Design review of the part built by this model. Coordinates are the model's own, in mm. Round coordinates to 2 decimals unless told otherwise and drop trailing zeros. Write each loop counter-clockwise with the first axis right and the second up, starting at its lowest first coordinate (ties: lowest second). Pieces come first, ordered by that corner, then holes. Notation, with made-up numbers: (-33.75, -40) -> (-22.75, -40) arc R13 cw to (-22.75, -26) -> close; hole circle Ø1 at (40.5, 79). An arc over 180 degrees is marked (long way). Write item = value, one per line. Start each with the question number.
Item 1: To check wall thickness, follow L1, parallel to Y at x = 12.5, z = 0.2; L2, parallel to Y at x = 10, z = 0.45; L3, parallel to Y at x = 14, z = 0.3. State the ranges of each line that lie inside material, in increasing order.
Item 2: Add section C-C, the plane x = 18.5. State the section outline as (y, z) points, then the cut area to 3 significant figures.
Item 3: Add section D-D, the plane y = -52. State the section outline as (x, z) points.
Item 4: Add section B-B, the plane y = 0. State the section outline as (x, z) points.
Item 5: Add section A-A, the plane z = 0.3. State how many separate pieces and enclosed holes the cut face has, then the cut area to 3 significant figures.
Item 6: For pin 1 Ø1 at (y, z) = (-20, 2) entering from -X; pin 2 Ø0.6 at (x, z) = (19, 0.5) entering from -Y; pin 3 Ø0.6 at (x, z) = (-10, 1) entering from -Y, all flat-tipped, find the tip position at first contact; note any pin that passes through.
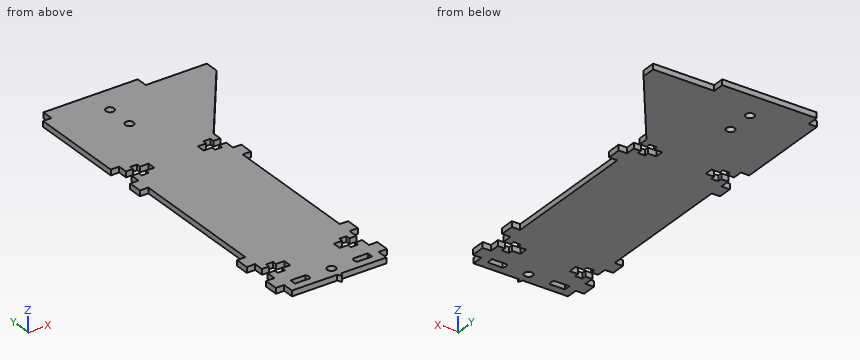
from build123d import *

# Parameters (mm, degrees)
SKETCH_1_R      = 1.5
EXTRUDE_1_DEPTH = 2


with BuildPart() as part:
    # 草图1 → 凸台-拉伸1 (new body)
    with BuildSketch(Plane.XY):
        Polygon((16.993865071, -34), (16.993865071, -84), (19.993865071, -84), (19.993865071, -89), (16.993865071, -89), (16.993865071, -92.5), (14.493865071, -92.5), (14.493865071, -91), (11.893865071, -91), (11.893865071, -92.5), (8.893865071, -92.5), (8.893865071, -95.5), (11.893865071, -95.5), (11.893865071, -97), (14.493865071, -97), (14.493865071, -95.5), (16.993865071, -95.5), (16.993865071, -99), (19.993865071, -99), (19.993865071, -104), (16.993865071, -104), (16.993865071, -108), (0.721190694, -108), (0, -109.5), (-0.721190694, -108), (-16.993865071, -108), (-16.993865071, -104), (-19.993865071, -104), (-19.993865071, -99), (-16.993865071, -99), (-16.993865071, -95.5), (-14.493865071, -95.5), (-14.493865071, -97), (-11.893865071, -97), (-11.893865071, -95.5), (-8.893865071, -95.5), (-8.893865071, -92.5), (-11.893865071, -92.5), (-11.893865071, -91), (-14.493865071, -91), (-14.493865071, -92.5), (-16.993865071, -92.5), (-16.993865071, -89), (-19.993865071, -89), (-19.993865071, -84), (-16.993865071, -84), (-16.993865071, -34), (-19.993865071, -34), (-19.993865071, -29), (-16.993865071, -29), (-16.993865071, -25.5), (-14.493865071, -25.5), (-14.493865071, -27), (-11.893865071, -27), (-11.893865071, -25.5), (-8.893865071, -25.5), (-8.893865071, -22.5), (-11.893865071, -22.5), (-11.893865071, -21), (-14.493865071, -21), (-14.493865071, -22.5), (-16.993865071, -22.5), (-16.993865071, -19), (-19.993865071, -19), (-19.993865071, 15.9), (-16.993865071, 15.9), (-16.993865071, 20), (16.993865071, 20), (16.993865071, 15.9), (38.993865071, 15.9), (38.993865071, 11), (16.993865071, -19), (16.993865071, -22.5), (14.493865071, -22.5), (14.493865071, -21), (11.893865071, -21), (11.893865071, -22.5), (8.893865071, -22.5), (8.893865071, -25.5), (11.893865071, -25.5), (11.893865071, -27), (14.493865071, -27), (14.493865071, -25.5), (16.993865071, -25.5), (16.993865071, -29), (19.993865071, -29), (19.993865071, -34), align=None)
        with Locations((0, -104)):
            Circle(SKETCH_1_R, mode=Mode.SUBTRACT)
        Circle(SKETCH_1_R, mode=Mode.SUBTRACT)
        with Locations((0, 10)):
            Circle(SKETCH_1_R, mode=Mode.SUBTRACT)
        with BuildLine():
            Line((13.9, -105.15), (8.6, -105.15))
            ThreePointArc((8.6, -105.15), (8.123654403, -104), (8.6, -102.85))
            Line((8.6, -102.85), (13.9, -102.85))
            Line((13.9, -102.85), (13.9, -105.15))
        make_face(mode=Mode.SUBTRACT)
        with BuildLine():
            Line((-13.9, -102.85), (-8.6, -102.85))
            ThreePointArc((-8.6, -102.85), (-8.123654403, -104), (-8.6, -105.15))
            Line((-8.6, -105.15), (-13.9, -105.15))
            Line((-13.9, -105.15), (-13.9, -102.85))
        make_face(mode=Mode.SUBTRACT)
    extrude(amount=EXTRUDE_1_DEPTH)


solid = part.part
Result set:
q1.L1 = -108 to -105.15, -102.85 to -97, -91 to -27, -21 to 20
q1.L2 = -108 to -105.15, -102.85 to -95.5, -92.5 to -25.5, -22.5 to 20
q1.L3 = -108 to -97, -91 to -27, -21 to 20
q2.outline = (-104, 0) -> (-99, 0) -> (-99, 2) -> (-104, 2) -> close; (-89, 0) -> (-84, 0) -> (-84, 2) -> (-89, 2) -> close; (-34, 0) -> (-29, 0) -> (-29, 2) -> (-34, 2) -> close; (-16.95, 0) -> (15.9, 0) -> (15.9, 2) -> (-16.95, 2) -> close
q2.area = 95.7 mm²
q3.outline = (-16.99, 0) -> (16.99, 0) -> (16.99, 2) -> (-16.99, 2) -> close
q4.outline = (-19.99, 0) -> (-1.5, 0) -> (-1.5, 2) -> (-19.99, 2) -> close; (1.5, 0) -> (30.93, 0) -> (30.93, 2) -> (1.5, 2) -> close
q5.separate_pieces = 1
q5.enclosed_holes = 5
q5.area = 4,810 mm²
q6.pin_1 = -16.99
q6.pin_2 = -104
q6.pin_3 = -108
